Geometry check sheet. Reference: the model listing, model coordinates, mm. Face numbers are marked on the shaded views. A direction names the side the tool comes from. Coordinates: 2 decimals unless noted, no trailing zeros. Order: outer loops, then holes, each group sorted by start corner. A loop starts at its lowest first (then second) coordinate and runs counter-clockwise, first axis right, second up. Notation, with made-up numbers: (71.25, -18.75) - (129.25, -18.75) arc R12 ccw to (129.25, 0.25) - close; hole circle Ø1 at (20, 14). An arc over 180 degrees is marked (long way). One line per item, written item: value. Start each with the question number.
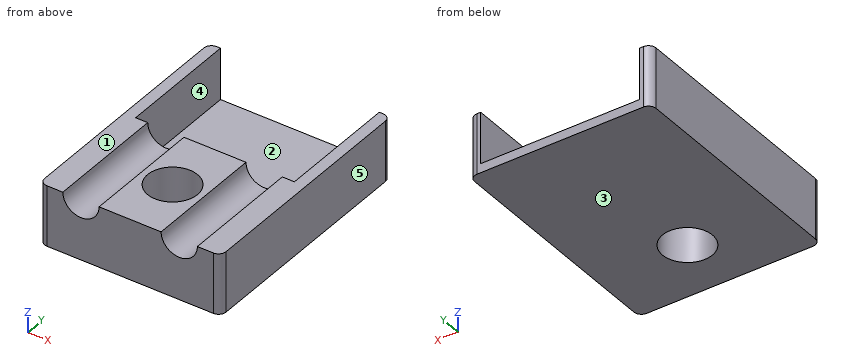
```python
from build123d import *

# Parameters (mm, degrees)
SKETCH1_R           = 1.65
BOSS_EXTRUDE1_DEPTH = 4
CUT_EXTRUDE1_DEPTH  = 16
SKETCH3_W           = 10.5
SKETCH3_H           = 3.4
CUT_EXTRUDE2_DEPTH  = 8


with BuildPart() as part:
    # Sketch1 → Boss-Extrude1 (new body)
    with BuildSketch(Plane.XY):
        with BuildLine():
            Line((0.5, 0), (11.5, 0))
            ThreePointArc((11.5, 0), (11.853553391, 0.146446609), (12, 0.5))
            Line((12, 0.5), (12, 15.5))
            ThreePointArc((12, 15.5), (11.853553391, 15.853553391), (11.5, 16))
            Line((11.5, 16), (0.5, 16))
            ThreePointArc((0.5, 16), (0.146446609, 15.853553391), (0, 15.5))
            Line((0, 15.5), (0, 0.5))
            ThreePointArc((0, 0.5), (0.146446609, 0.146446609), (0.5, 0))
        make_face()
        with Locations((6, 4)):
            Circle(SKETCH1_R, mode=Mode.SUBTRACT)
    extrude(amount=BOSS_EXTRUDE1_DEPTH)

    # Sketch2 → Cut-Extrude1 (cut)
    with BuildSketch(Plane.XZ):
        with BuildLine():
            Line((1.55, 4), (3.95, 4))
            ThreePointArc((3.95, 4), (2.75, 2.8), (1.55, 4))
        make_face()
        with BuildLine():
            Line((8.05, 4), (10.45, 4))
            ThreePointArc((10.45, 4), (9.25, 2.8), (8.05, 4))
        make_face()
    extrude(amount=-CUT_EXTRUDE1_DEPTH, mode=Mode.SUBTRACT)

    # Sketch3 → Cut-Extrude2 (cut)
    with BuildSketch(Plane(origin=(0, 16, 0), x_dir=(1, 0, 0), z_dir=(0, 1, 0))):
        with Locations((6, -2.3)):
            Rectangle(SKETCH3_W, SKETCH3_H)
    extrude(amount=-CUT_EXTRUDE2_DEPTH, mode=Mode.SUBTRACT)


solid = part.part
```
Q1. Cross-section at B-B, the plane x = 6. Enter the section's corners in (y, z).
Q2. Release check for a two-part mould opening along X. For the marked faces 3, 4 and 5 record: released by +X, released by -X, zero draft, split by the parting line, or undercut.
Q3. Cross-section at C-C, the plane y = 4. Enter the section's corners in (x, z), and give its area (3 significant figures).
Q4. Cross-section at A-A, the plane z = 2.6. Enter the section's corners in (x, y), and give its area (3 significant figures).
Q5. Set-up check for the marked faces 1 and 2: record each of +Z, -Z, +X, -X, +Y, -Y from which the full face is reachable in a straight line by a thin tool's end or side.
Q6. Cross-section at D-D, the plane z = 3.65. Enter the section's corners in (x, y), and give its area (3 significant figures).
Q7. Material ranges on probe 1 along X at (y, z) = (9.5, 1.9); probe 2 along Y at (x, z) = (6, 2.3); probe 3 along Y at (x, z) = (1.25, 3.45), recorded low to high.
Q8. Gauge pin test, flat ends, axial feed: P1, Ø3, axis at x = 6, y = 4, coming from the +Z side; P2, Ø1.5, axis at x = 3, z = 3, coming from the +Y side. Record the tip position at first contact, or that the pin passes through.
Check result:
1. outline: (0, 0) - (2.35, 0) - (2.35, 4) - (0, 4) - close; (5.65, 0) - (16, 0) - (16, 0.6) - (8, 0.6) - (8, 4) - (5.65, 4) - close
2. face 3: zero draft
2. face 4: undercut
2. face 5: released by +X
3. outline: (0, 0) - (4.35, 0) - (4.35, 4) - (3.95, 4) arc R1.2 cw to (1.55, 4) - (0, 4) - close; (7.65, 0) - (12, 0) - (12, 4) - (10.45, 4) arc R1.2 cw to (8.05, 4) - (7.65, 4) - close
3. area: 30.3 mm2
4. outline: (0, 0.5) arc R0.5 ccw to (0.5, 0) - (11.5, 0) arc R0.5 ccw to (12, 0.5) - (12, 15.5) arc R0.5 ccw to (11.5, 16) - (11.25, 16) - (11.25, 8) - (0.75, 8) - (0.75, 16) - (0.5, 16) arc R0.5 ccw to (0, 15.5) - close; hole circle Ø3.3 at (6, 4)
4. area: 99.2 mm2
5. face 1: +Z, +X, -X, +Y, -Y
5. face 2: +Z, +Y
6. outline: (0, 0.5) arc R0.5 ccw to (0.5, 0) - (1.6, 0) - (1.6, 8) - (0.75, 8) - (0.75, 16) - (0.5, 16) arc R0.5 ccw to (0, 15.5) - close; (3.9, 0) - (8.1, 0) - (8.1, 8) - (3.9, 8) - close; (10.4, 0) - (11.5, 0) arc R0.5 ccw to (12, 0.5) - (12, 15.5) arc R0.5 ccw to (11.5, 16) - (11.25, 16) - (11.25, 8) - (10.4, 8) - close; hole circle Ø3.3 at (6, 4)
6. area: 62.5 mm2
7. probe 1: x = 0 to 0.75, 11.25 to 12
7. probe 2: y = 0 to 2.35, 5.65 to 8
7. probe 3: y = 0 to 8
8. P1: passes through
8. P2: stops at y = 8
